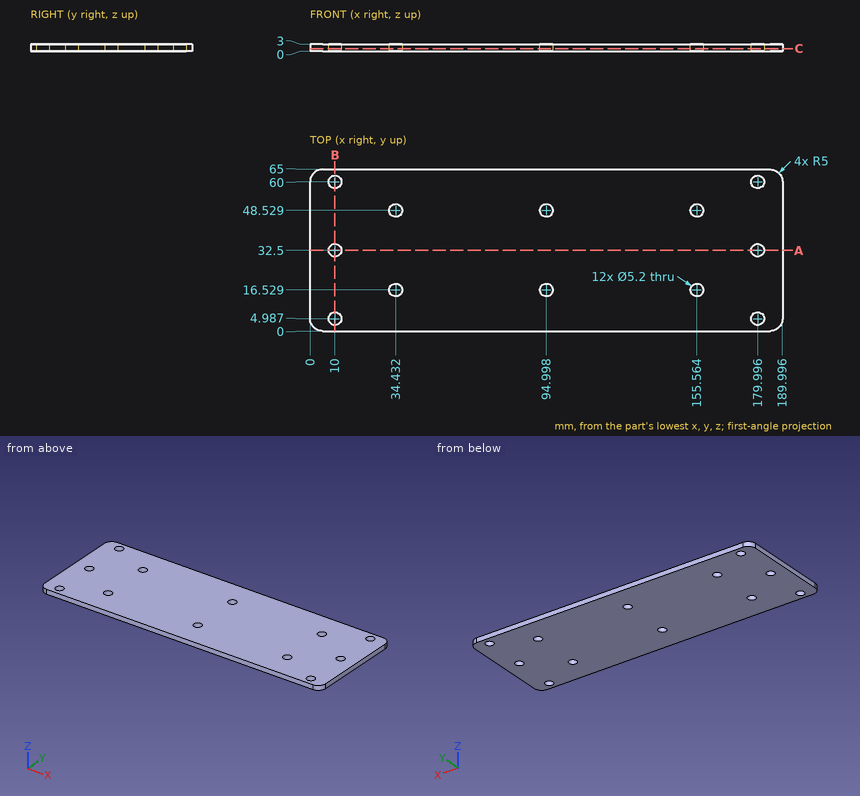
Could you check a few things on this drawing? It's one solid part, dimensions in mm from its lowest x, y, z. Round coordinates to 2 decimals unless told otherwise and drop trailing zeros. Loops run counter-clockwise (first coordinate to the right, second up) from the corner with the lowest first, then second, coordinate; pieces in that order, holes last. Notation, with made-up numbers: M -22.5,34 L 8.5,34 A14 ccw 8.5,44 Z; hole C 42.5,11 d4. An arc over 180 degrees is marked long. Write item = value, one per line. Start each with the question number.
(1) Suppose I cut it at B-B on x = 10. Write out the boundary of the cut face in (y, z).
(2) Suppose I cut it at C-C on z = 1.15. Give the number of separate pieces and of enclosed holes in the cut face, plus the area to 3 significant figures.
(3) Suppose I cut it at A-A on y = 32.5. Write out the boundary of the cut face in (x, z), plus the area to 3 significant figures.
(4) I need wall thicknesses on line 1 along Y through (x, z) = (10, 1.25); line 2 along X through (y, z) = (61, 2.6) (1 decimal); line 3 along Y through (x, z) = (153.5, 1.85). Which ranges of each line are inside material? Lowest first, please.
Answer block:
q1.outline = M 0,0 L 2.39,0 L 2.39,3 L 0,3 Z; M 7.59,0 L 29.9,0 L 29.9,3 L 7.59,3 Z; M 35.1,0 L 57.4,0 L 57.4,3 L 35.1,3 Z; M 62.6,0 L 65,0 L 65,3 L 62.6,3 Z
q2.separate_pieces = 1
q2.enclosed_holes = 12
q2.area = 12,100 mm²
q3.outline = M 0,0 L 7.4,0 L 7.4,3 L 0,3 Z; M 12.6,0 L 177.4,0 L 177.4,3 L 12.6,3 Z; M 182.6,0 L 190,0 L 190,3 L 182.6,3 Z
q3.area = 539 mm²
q4.line_1 = 0 to 2.39, 7.59 to 29.9, 35.1 to 57.4, 62.6 to 65
q4.line_2 = 0.1 to 7.6, 12.4 to 177.6, 182.4 to 189.9
q4.line_3 = 0 to 14.95, 18.11 to 46.95, 50.11 to 65
